```python
from build123d import *

# Parameters (mm, degrees)
SKETCH_1_R      = 1.5
SKETCH_1_R_2    = 2.1
SKETCH_1_R_3    = 25
SKETCH_1_R_4    = 2
SKETCH_1_W      = 4.3
SKETCH_1_H      = 8.3
EXTRUDE_1_DEPTH = 4
FILLET_1_R      = 2


with BuildPart() as part:
    # 草图1 → 凸台-拉伸1 (new body)
    with BuildSketch(Plane.XY):
        with BuildLine():
            Line((-54, 52.4), (-54, -52.5))
            Line((-54, -52.5), (54, -52.5))
            Line((54, -52.5), (54, 52.4))
            ThreePointArc((54, 52.4), (33.845954515, 70.803240423), (8, 79.569735886))
            Line((8, 79.569735886), (8, 90.5))
            Line((8, 90.5), (28, 90.5))
            Line((28, 90.5), (28, 106.5))
            Line((28, 106.5), (-28, 106.5))
            Line((-28, 106.5), (-28, 90.5))
            Line((-28, 90.5), (-8, 90.5))
            Line((-8, 90.5), (-8, 79.569735886))
            ThreePointArc((-8, 79.569735886), (-33.845954515, 70.803240423), (-54, 52.4))
        make_face()
        with Locations((-47, 37.5)):
            Circle(SKETCH_1_R, mode=Mode.SUBTRACT)
        with Locations((-47, 7.5)):
            Circle(SKETCH_1_R, mode=Mode.SUBTRACT)
        with Locations((-47, -22.5)):
            Circle(SKETCH_1_R, mode=Mode.SUBTRACT)
        with Locations((-23.57, 37.07)):
            Circle(SKETCH_1_R_2, mode=Mode.SUBTRACT)
        with Locations((-23.57, -10.07)):
            Circle(SKETCH_1_R_2, mode=Mode.SUBTRACT)
        with Locations((23.57, -10.07)):
            Circle(SKETCH_1_R_2, mode=Mode.SUBTRACT)
        with Locations((23.57, 37.07)):
            Circle(SKETCH_1_R_2, mode=Mode.SUBTRACT)
        with Locations((47, -22.5)):
            Circle(SKETCH_1_R, mode=Mode.SUBTRACT)
        with Locations((47, 7.5)):
            Circle(SKETCH_1_R, mode=Mode.SUBTRACT)
        with Locations((47, 37.5)):
            Circle(SKETCH_1_R, mode=Mode.SUBTRACT)
        with Locations((0, 13.5)):
            Circle(SKETCH_1_R_3, mode=Mode.SUBTRACT)
        with Locations((0, 60.5)):
            Circle(SKETCH_1_R_4, mode=Mode.SUBTRACT)
        with Locations((33.234018716, 46.734018716)):
            Circle(SKETCH_1_R_4, mode=Mode.SUBTRACT)
        with Locations((33.234018716, -19.734018716)):
            Circle(SKETCH_1_R_4, mode=Mode.SUBTRACT)
        with Locations((0, -33.5)):
            Circle(SKETCH_1_R_4, mode=Mode.SUBTRACT)
        with Locations((-33.234018716, -19.734018716)):
            Circle(SKETCH_1_R_4, mode=Mode.SUBTRACT)
        with Locations((-33.234018716, 46.734018716)):
            Circle(SKETCH_1_R_4, mode=Mode.SUBTRACT)
        with Locations((0, 78.5)):
            Circle(SKETCH_1_R_4, mode=Mode.SUBTRACT)
        with Locations((-20, 98.5)):
            Circle(SKETCH_1_R_4, mode=Mode.SUBTRACT)
        with Locations((20, 98.5)):
            Circle(SKETCH_1_R_4, mode=Mode.SUBTRACT)
        with Locations((-47, 22.5)):
            Rectangle(SKETCH_1_W, SKETCH_1_H, mode=Mode.SUBTRACT)
        with Locations((-47, -7.5)):
            Rectangle(SKETCH_1_W, SKETCH_1_H, mode=Mode.SUBTRACT)
        with Locations((-47, -37.5)):
            Rectangle(SKETCH_1_W, SKETCH_1_H, mode=Mode.SUBTRACT)
        with Locations((47, -37.5)):
            Rectangle(SKETCH_1_W, SKETCH_1_H, mode=Mode.SUBTRACT)
        with Locations((47, -7.5)):
            Rectangle(SKETCH_1_W, SKETCH_1_H, mode=Mode.SUBTRACT)
        with Locations((47, 22.5)):
            Rectangle(SKETCH_1_W, SKETCH_1_H, mode=Mode.SUBTRACT)
    extrude(amount=EXTRUDE_1_DEPTH)

    # 圆角1
    fillet_1_edges = [part.edges().sort_by_distance(p)[0] for p in [
        (-8, 79.569735886, 2),
        (-8, 90.5, 2),
        (-28, 90.5, 2),
        (-28, 106.5, 2),
        (28, 106.5, 2),
        (28, 90.5, 2),
        (8, 90.5, 2),
        (8, 79.569735886, 2),
    ]]
    fillet(fillet_1_edges, radius=FILLET_1_R)


solid = part.part
```
Input: part model. Units: mm. Frame: model coordinates. A direction names the side the tool comes from. Round coordinates to 2 decimals unless told otherwise and drop trailing zeros. Order: outer loops, then holes, each group sorted by start corner. A loop starts at its lowest first (then second) coordinate and runs counter-clockwise, first axis right, second up. Notation, with made-up numbers: (-36.75, 36) - (13.25, 36) arc R19 ccw to (13.25, 63) - close; hole circle Ø7 at (10.5, -24). An arc over 180 degrees is marked (long way). One line per question, with ' | ' between items. Start each with the question number.
1) Cut plane B-B, the plane y = 24.5. Return the cut outline in (x, z).
2) Ray query, probe 1 along X at (y, z) = (-41, 1.9); probe 2 along Y at (x, z) = (0, 2.95); probe 3 along Y at (x, z) = (45, 2.3). Return the intervals inside material, ascending.
3) Set-up query: faces 4 (the flat face through (-49.15, 22, 2)), 5 (the flat face through (0, 106.5, 2)), 6 (the flat face through (18, 90.5, 2)). Return all of +Z, -Z, +X, -X, +Y, -Y with unobstructed straight access to the full face (end or side cutting, diameter ignored); none if empty.
4) Cut plane A-A, the plane y = 60.5. Return the cut outline in (x, z).
5) Cut plane D-D, the plane x = -42.5. Return the cut outline in (y, z).
6) Pull-direction query (X, two-part tool) for faces 1 (the flat face through (-8, 85, 2)), 2 (the flat face through (23, 28, 4)), 3 (the flat face through (-47, 18.35, 2)); classes: +X half, -X half, draft (parallel to the pull), parting line (faces both ways), or undercut.
7) Cut plane C-C, the plane x = 15.5. Return the cut outline in (y, z), then the cut area to 3 significant figures.
8) Contact query for flat-ended pins moving along their axis: P1, Ø1.5, axis at x = 5.5, y = 59, coming from the -Z side; P2, Ø1.2, axis at x = -46.5, z = 3, coming from the +Y side; P3, Ø2, axis at y = 74, z = 0.5, coming from the -X side; P4, Ø2, axis at x = 48, z = 1, coming from the +Y side. Output: stop coordinate, or through.
Worked out:
1) outline: (-54, 0) - (-49.15, 0) - (-49.15, 4) - (-54, 4) - close; (-44.85, 0) - (-22.45, 0) - (-22.45, 4) - (-44.85, 4) - close; (22.45, 0) - (44.85, 0) - (44.85, 4) - (22.45, 4) - close; (49.15, 0) - (54, 0) - (54, 4) - (49.15, 4) - close
2) probe 1: x = -54 to -49.15, -44.85 to 44.85, 49.15 to 54 | probe 2: y = -52.5 to -35.5, -31.5 to -11.5, 38.5 to 58.5, 62.5 to 76.5, 80.5 to 106.5 | probe 3: y = -52.5 to -41.65, -33.35 to -11.65, -3.35 to 18.35, 26.65 to 62.53
3) face 4: +Z, -Z | face 5: +Z, -Z, +X, -X, +Y | face 6: +Z, -Z, +X
4) outline: (-47.12, 0) - (-2, 0) - (-2, 4) - (-47.12, 4) - close; (2, 0) - (47.12, 0) - (47.12, 4) - (2, 4) - close
5) outline: (-52.5, 0) - (64.71, 0) - (64.71, 4) - (-52.5, 4) - close
6) face 1: -X half | face 2: draft | face 3: undercut
7) outline: (-52.5, 0) - (-6.12, 0) - (-6.12, 4) - (-52.5, 4) - close; (33.12, 0) - (78.22, 0) - (78.22, 4) - (33.12, 4) - close; (90.5, 0) - (106.5, 0) - (106.5, 4) - (90.5, 4) - close | area: 430 mm^2
8) P1: stops at z = 0 | P2: stops at y = 61.69 | P3: stops at x = -29.82 | P4: stops at y = 60.62
